Here's how the part is built. I have some questions about the finished solid (model axes, mm). Face numbers are marked on the shaded views. A direction names the side the tool comes from. Round coordinates to 2 decimals unless told otherwise and drop trailing zeros. Loops run counter-clockwise (first coordinate to the right, second up) from the corner with the lowest first, then second, coordinate; pieces in that order, holes last. Notation, with made-up numbers: M 18,7 L 42,7 A14 cw 42,22 Z; hole C 41,83 d1. An arc over 180 degrees is marked long. Write item = value, one per line. Start each with the question number.
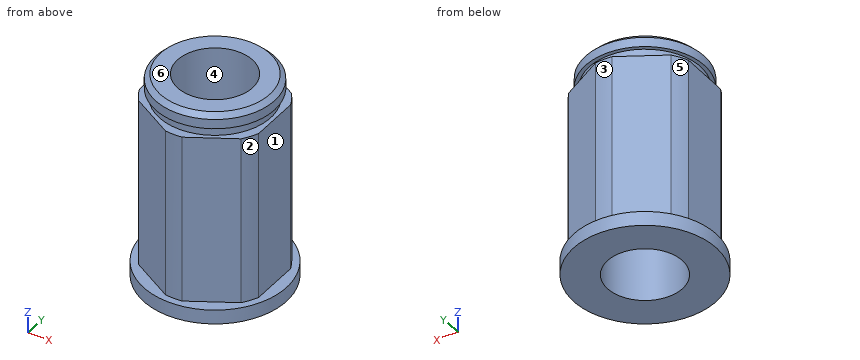
from build123d import *

# Parameters (mm, degrees)
SKETCH1_R               = 6.35
BASIC_ROD_DEPTH         = 9.779
BASIC_ROD_DEPTH_BACK    = 9.779
THEX_DEPTH              = 9.779
SKETCH2_R               = 4.0005
INTERNAL_CUT_DEPTH      = 13.319
INTERNAL_CUT_DEPTH_BACK = 10.779
SKETCH9_R               = 7.62
SKETCH9_R_2             = 4.0005
BOSS_EXTRUDE1_DEPTH     = 1.524


with BuildPart() as part:
    # Sketch1 → Basic Rod (new body, two sides)
    with BuildSketch(Plane.XY) as basic_rod_sk:
        Circle(SKETCH1_R)
    extrude(amount=BASIC_ROD_DEPTH)
    extrude(basic_rod_sk.sketch, amount=-BASIC_ROD_DEPTH_BACK)

    # Sketch8 → THex (add, symmetric)
    with BuildSketch(Plane.XY):
        with BuildLine():
            Line((-0.888411378, 6.819423871), (-5.461588622, 4.179098758))
            ThreePointArc((-5.461588622, 4.179098758), (-5.955700003, 3.438525), (-6.35, 2.640325113))
            Line((-6.35, 2.640325113), (-6.35, -2.640325113))
            ThreePointArc((-6.35, -2.640325113), (-5.955700003, -3.438525), (-5.461588622, -4.179098758))
            Line((-5.461588622, -4.179098758), (-0.888411378, -6.819423871))
            ThreePointArc((-0.888411378, -6.819423871), (0, -6.87705), (0.888411378, -6.819423871))
            Line((0.888411378, -6.819423871), (5.461588622, -4.179098758))
            ThreePointArc((5.461588622, -4.179098758), (5.955700003, -3.438525), (6.35, -2.640325113))
            Line((6.35, -2.640325113), (6.35, 2.640325113))
            ThreePointArc((6.35, 2.640325113), (5.955700003, 3.438525), (5.461588622, 4.179098758))
            Line((5.461588622, 4.179098758), (0.888411378, 6.819423871))
            ThreePointArc((0.888411378, 6.819423871), (0, 6.87705), (-0.888411378, 6.819423871))
        make_face()
    extrude(amount=THEX_DEPTH, both=True)

    # Sketch7 → 1stSnapRing (revolve)
    with BuildSketch(Plane(origin=(0, 0, 0), x_dir=(0, 0, -1), z_dir=(1, 0, 0))):
        Polygon((-9.779, 5.9436), (-10.795, 5.9436), (-10.795, 6.35), (-11.811, 6.35), (-12.319, 5.842), (-12.319, 0), (-9.779, 0), align=None)
    revolve(axis=Axis((0, 0, -38.2778), (0, 0, 1)))

    # Sketch2 → Internal Cut (cut, two sides)
    with BuildSketch(Plane.XY) as internal_cut_sk:
        Circle(SKETCH2_R)
    extrude(amount=INTERNAL_CUT_DEPTH, mode=Mode.SUBTRACT)
    extrude(internal_cut_sk.sketch, amount=-INTERNAL_CUT_DEPTH_BACK, mode=Mode.SUBTRACT)

    # Sketch9 → Boss-Extrude1 (add)
    with BuildSketch(Plane(origin=(0, 0, -9.779), x_dir=(-1, 0, 0), z_dir=(0, 0, -1))):
        Circle(SKETCH9_R)
        Circle(SKETCH9_R_2, mode=Mode.SUBTRACT)
    extrude(amount=-BOSS_EXTRUDE1_DEPTH)


solid = part.part
Item 1: For the marked faces 1, 2 and 3, which set-ups out of +Z, -Z, +X, -X, +Y, -Y let a thin tool reach every point of the face, with its end or its side?
Item 2: Will these pins go through, and if not, where does the flat tip stop? pin 1 Ø6 at (y, z) = (2.5, 9) entering from +X; pin 2 Ø6.5 at (x, y) = (0, 2) entering from +Z; pin 3 Ø2 at (y, z) = (-2.5, 1.5) entering from -X; pin 4 Ø2 at (y, z) = (4, -3) entering from -X.
Item 3: I want a section at C-C, the plane z = -3.5. List the corners of the cut face in (x, y) for me, then the cut area to 3 significant figures.
Item 4: We'd pull the mould along X, two halves only. Please class the marked faces 4, 5 and 6: released by +X, released by -X, zero draft, split by the parting line, or undercut.
Item 5: Please list where these lines run through material, in increasing order: line 1 (X direction, y = 0, z = 3); line 2 (Y direction, x = 0, z = 0.25); line 3 (Z direction, x = -4, y = -5.75) (3 decimals). Write a range as [from, to].
Worked out:
q1.face_1 = +Z, +X, +Y, -Y
q1.face_2 = +Z, +X, -Y
q1.face_3 = +Z, +Y
q2.pin_1 = 6.35
q2.pin_2 = 12.32
q2.pin_3 = -6.35
q2.pin_4 = -6.19
q3.outline = M -6.35,-2.64 A6.88 ccw -5.46,-4.18 L -0.89,-6.82 A6.88 ccw 0.89,-6.82 L 5.46,-4.18 A6.88 ccw 6.35,-2.64 L 6.35,2.64 A6.88 ccw 5.46,4.18 L 0.89,6.82 A6.88 ccw -0.89,6.82 L -5.46,4.18 A6.88 ccw -6.35,2.64 Z; hole C 0,0 d8
q3.area = 87.1 mm2
q4.face_4 = undercut
q4.face_5 = released by -X
q4.face_6 = zero draft
q5.line_1 = [-6.35, -4], [4, 6.35]
q5.line_2 = [-6.88, -4], [4, 6.88]
q5.line_3 = [-9.779, -8.255]
